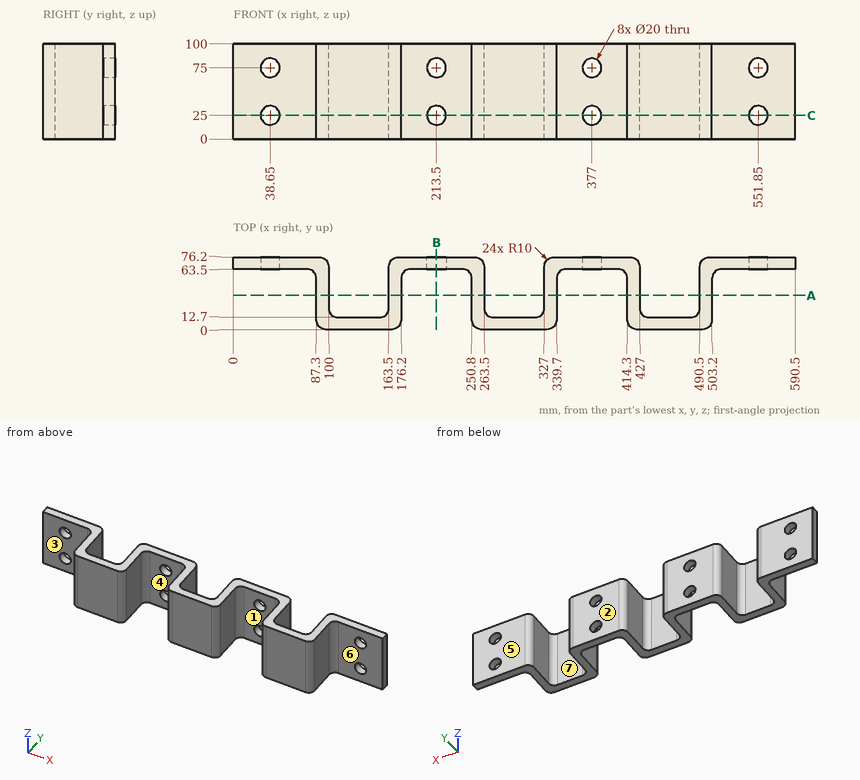
Answer from the drawing. Dimensions are ordinates in mm from the lowest x, y and z of the part. A direction names the side the tool comes from. Coordinates: 2 decimals unless noted, no trailing zeros. Write each loop counter-clockwise with the first axis right and the second up, starting at its lowest first coordinate (ties: lowest second). Pieces come first, ordered by that corner, then holes. Notation, with made-up numbers: (31.25, -3) - (51.25, -3) arc R18 ccw to (51.25, 26) - close; hole circle Ø6 at (55.5, 48). An arc over 180 degrees is marked (long way). Return JSON: item names as keys, results as strings. Group by question number.
Q1. Flat-ended cylindrical pins translate along their axes: pin 1 Ø3 at (y, z) = (60.5, 66) entering from -X; pin 2 Ø22 at (y, z) = (34, 30) entering from -X; pin 3 Ø13 at (x, z) = (122.5, 50) entering from +Y. Find the tip coordinate at first contact, or state that the pin passes through.
Q2. The part is cut by section A-A on y = 36. Write down the section's boundary in (x, z), and give its area (3 significant figures).
Q3. For a pull along X with two mould halves and no side action, classify the marked faces 1 and 2 as +X half, -X half, draft (parallel to the pull), parting line (faces both ways), or undercut.
Q4. Which of the six approach directions +Z, -Z, +X, -X, +Y, -Y give full straight-line access (tool end or side, diameter ignored) to the marked faces 3, 4, 5, 6 and 7?
Q5. The part is cut by section C-C on z = 25. State how many separate pieces and enclosed holes the cut face has, and give its area (3 significant figures).
Q6. Find the intervals of material crossed by line 1 along Z through (x, y) = (551, 70); line 2 along X through (y, z) = (36, 50.5); line 3 along Y through (x, z) = (72, 9), in increasing order. Write a range as [from, to].
Q7. The part is cut by section B-B on x = 213.5. Write down the section's boundary in (y, z).
Evaluation:
{
 "1": {"pin 1": "stops at x = 82.57", "pin 2": "stops at x = 87.3", "pin 3": "stops at y = 12.7"},
 "2": {"outline": "(87.3, 0) - (100, 0) - (100, 100) - (87.3, 100) - close; (163.5, 0) - (176.2, 0) - (176.2, 100) - (163.5, 100) - close; (250.8, 0) - (263.5, 0) - (263.5, 100) - (250.8, 100) - close; (327, 0) - (339.7, 0) - (339.7, 100) - (327, 100) - close; (414.3, 0) - (427, 0) - (427, 100) - (414.3, 100) - close; (490.5, 0) - (503.2, 0) - (503.2, 100) - (490.5, 100) - close", "area": "7,620 mm2"},
 "3": {"face 1": "undercut", "face 2": "draft"},
 "4": {"face 3": "+Z, -Z, -X, -Y", "face 4": "+Z, -Z, -Y", "face 5": "+Z, -Z, +X, -X, +Y", "face 6": "+Z, -Z, +X, -Y", "face 7": "+Z, -Z, +Y"},
 "5": {"separate pieces": "5", "enclosed holes": "0", "area": "11,300 mm2"},
 "6": {"line 1": "z = [0, 15.04], [34.96, 65.04], [84.96, 100]", "line 2": "x = [87.3, 100], [163.5, 176.2], [250.8, 263.5], [327, 339.7], [414.3, 427], [490.5, 503.2]", "line 3": "y = [63.5, 76.2]"},
 "7": {"outline": "(63.5, 0) - (76.2, 0) - (76.2, 15) - (63.5, 15) - close; (63.5, 35) - (76.2, 35) - (76.2, 65) - (63.5, 65) - close; (63.5, 85) - (76.2, 85) - (76.2, 100) - (63.5, 100) - close"}
}
